Solid Edge part; units mm, degrees
sketch "Sketch1" plane through (0, 0, 0) normal (0, 0, 1) x (1, 0, 0)
  line L0 (-17.5, 30) -> (17.5, 30)
  line L1 (17.5, 30) -> (17.5, 15)
  line L2 (17.5, 15) -> (22.3, 15)
  line L3 (22.3, 0) -> (22.3, 15)
  line L4 (22.3, 0) -> (22.3, -15)
  line L5 (22.3, -15) -> (17.5, -15)
  line L6 (17.5, -30) -> (17.5, -15)
  line L7 (-17.5, -30) -> (17.5, -30)
  line L8 (-17.5, -15) -> (-17.5, -30)
  line L9 (-22.3, -15) -> (-17.5, -15)
  line L10 (-22.3, 0) -> (-22.3, -15)
  line L11 (-22.3, 0) -> (-22.3, 15)
  line L12 (-17.5, 15) -> (-22.3, 15)
  line L13 (-17.5, 15) -> (-17.5, 30)
  circle A0 centre (3.45, 14.41) radius 1.25
  circle A1 centre (-7.895, 10.99) radius 1.25
  circle A2 centre (-3.45, -14.41) radius 1.25
  circle A3 centre (7.895, -10.99) radius 1.25
extrude "ExtrudedProtrusion_6" add sketch "Sketch1" along normal blind 4.8
sketch "Sketch2" plane through (0, 0, 4.8) normal (0, 0, 1) x (1, 0, 0)
  line L0 (-19.9, 15) -> (-19.9, -15.25)
  line L1 (-19.9, -15.25) -> (-17.5, -15.25)
  line L2 (-17.5, -15.25) -> (-17.5, 15)
  line L3 (-17.5, 15) -> (-19.9, 15)
  line L4 (19.9, -15) -> (19.9, 15)
  line L5 (19.9, 15) -> (17.5, 15)
  line L6 (17.5, 15) -> (17.5, -15)
  line L7 (17.5, -15) -> (19.9, -15)
extrude "ExtrudedCutout_5" cut sketch "Sketch2" against normal blind 2.4
sketch "Sketch3" plane through (0, -0.25, 4.8) normal (0, 0, 1) x (1, 0, 0)
  line L0 (6.2615, 8.9272) -> (-10.0146, 4.0193)
  arc A0 (-13.3582, -2.2113) -> (-10.0146, 4.0193) centre (-8.5711, -0.7678) cw
  line L1 (-13.3582, -2.2113) -> (-12.7808, -4.1261)
  arc A1 (-12.7808, -4.1261) -> (-6.5502, -7.4697) centre (-7.9937, -2.6826) ccw
  line L2 (-6.5502, -7.4697) -> (9.7259, -2.5619)
  arc A2 (9.7259, -2.5619) -> (13.0695, 3.6687) centre (8.2824, 2.2252) ccw
  line L3 (13.0695, 3.6687) -> (12.4921, 5.5835)
  arc A3 (6.2615, 8.9272) -> (12.4921, 5.5835) centre (7.705, 4.1401) cw
extrude "ExtrudedCutout_7" cut sketch "Sketch3" against normal blind 5
sketch "Sketch4" plane through (0, -0.25, 4.8) normal (0, 0, 1) x (1, 0, 0)
  arc A0 (-17.5, 18.25) -> (-17.5, 15.25) centre (-17.5, 16.75) cw
  line L0 (-17.5, 15.25) -> (-17.5, 18.25)
  arc A1 (-17.5, -14.75) -> (-17.5, -17.75) centre (-17.5, -16.25) cw
  line L1 (-17.5, -14.75) -> (-17.5, -17.75)
  arc A2 (17.5, -17.75) -> (17.5, -14.75) centre (17.5, -16.25) cw
  line L2 (17.5, -14.75) -> (17.5, -17.75)
  line L3 (17.5, 15.25) -> (17.5, 18.25)
  arc A3 (17.5, 15.25) -> (17.5, 18.25) centre (17.5, 16.75) cw
extrude "Cutout1" cut sketch "Sketch4" against normal blind 5
sketch "Sketch5" plane through (0, -0.25, 0) normal (0, 0, -1) x (-1, 0, 0)
  line L0 (-1.6, 30.25) -> (-1.6, 27.2024)
  arc A0 (-1.6, 27.2024) -> (-2.725, 25.75) centre (-1.225, 25.75) ccw
  line L1 (-2.725, 25.75) -> (-2.725, 24.25)
  arc A1 (-2.725, 24.25) -> (-1.5998, 22.7976) centre (-1.225, 24.25) ccw
  arc A2 (-1.5998, 22.7976) -> (1.5998, 22.7976) centre (0, 22.7754) ccw
  arc A3 (2.725, 24.25) -> (1.5998, 22.7976) centre (1.225, 24.25) cw
  line L2 (2.725, 25.75) -> (2.725, 24.25)
  arc A4 (1.5998, 27.2024) -> (2.725, 25.75) centre (1.225, 25.75) cw
  line L3 (1.5998, 30.25) -> (1.5998, 27.2024)
  line L4 (0, 30.25) -> (1.5998, 30.25)
  line L5 (0, 30.25) -> (-1.6, 30.25)
  arc A5 (-1.5998, -22.2976) -> (1.5998, -22.2976) centre (0, -22.2754) cw
  arc A6 (2.725, -23.75) -> (1.5998, -22.2976) centre (1.225, -23.75) ccw
  line L6 (2.725, -25.25) -> (2.725, -23.75)
  arc A7 (1.5998, -26.7024) -> (2.725, -25.25) centre (1.225, -25.25) ccw
  line L7 (1.5998, -29.75) -> (1.5998, -26.7024)
  line L8 (0, -29.75) -> (1.5998, -29.75)
  line L9 (0, -29.75) -> (-1.6, -29.75)
  line L10 (-1.6, -29.75) -> (-1.6, -26.7024)
  arc A8 (-1.6, -26.7024) -> (-2.725, -25.25) centre (-1.225, -25.25) cw
  line L11 (-2.725, -25.25) -> (-2.725, -23.75)
  arc A9 (-2.725, -23.75) -> (-1.5998, -22.2976) centre (-1.225, -23.75) cw
extrude "Cutout2" cut sketch "Sketch5" against normal up to next
properties material "Polycarbonate"
Here's how the part is built. I have some questions about the finished solid (model axes, mm). A direction names the side the tool comes from. Give positions to 0.01 mm unless a question says otherwise; leave off trailing zeros. Order: outer loops, then holes, each group sorted by start corner. A loop starts at its lowest first (then second) coordinate and runs counter-clockwise, first axis right, second up. Notation, with made-up numbers: (9, 68.25) -> (57, 68.25) arc R26 ccw to (57, 104.25) -> close; hole circle Ø5 at (28.25, 78.25). An arc over 180 degrees is marked (long way). Use a Markdown table: item, result. Add a question column.
Item 1: For faces 1 (the face through (-17.5, 0, 4)), 2 (the face through (-20, -15, 2)), 3 (the face through (-10, 30, 2)), 4 (the face through (0, -6, 4.8)), 5 (the face through (10.12, 8.27, 2.43)), which set-ups out of +Z, -Z, +X, -X, +Y, -Y let a thin tool reach every point of the face, with its end or its side?
Item 2: Imagine slicing it at B-B on z = 3.95. Give the number of separate pieces and of enclosed holes in the cut face, plus the area to 3 significant figures.
Item 3: I need wall thicknesses on line 1 (X direction, y = -24.5, z = 2) (3 decimals); line 2 (Y direction, x = 8.5, z = 3.75); line 3 (Y direction, x = -3.45, z = 2). Which ranges of each line are inside material? Lowest first, please.
Item 4: Imagine slicing it at A-A on y = -10.99. Please give me the cut outline in (x, z) (3 decimals), plus the area to 3 significant figures.
Item 5: Will these pins go through, and if not, where does the flat tip stop? pin 1 (3 mm diameter, centred on x = -3.45, y = -14.41, fed in from -Z); pin 2 (0.9 mm diameter, centred on y = -28, z = 1.5, fed in from +X); pin 3 (0.9 mm diameter, centred on y = 28, z = 3, fed in from -X).
Item 6: Imagine slicing it at D-D on x = 8. Please give me the cut outline in (y, z).
Item 7: Imagine slicing it at C-C on x = 0.5. Please give me the cut outline in (y, z).
Item 8: If we mould it in two halves opening along X, with no side actions, what happens to faces 6 (the face through (21, 0, 4.8)), 7 (the face through (-1.76, 6.26, 2.43)), 8 (the face through (16, 16.5, 2.4))? For each: pulls with the +X half, pulls with the -X half, needs draft (parallel to the pull), parting line crosses it, or undercut.
Data:
| question | item | result |
|---|---|---|
| 1 | face 1 | +Z, +Y, -Y |
| 1 | face 2 | +Z, -Z, -X, -Y |
| 1 | face 3 | +Z, -Z, +X, -X, +Y |
| 1 | face 4 | +Z, +X, -X, +Y, -Y |
| 1 | face 5 | +Z, -Z |
| 2 | separate pieces | 3 |
| 2 | enclosed holes | 5 |
| 2 | area | 1,840 mm² |
| 3 | line 1 | x = -17.5 to -2.725, 2.725 to 17.5 |
| 3 | line 2 | y = -30 to -12.08, -9.9 to -3.18, 8.83 to 30 |
| 3 | line 3 | y = -30 to -15.66, -13.16 to -6.78, 5.75 to 30 |
| 4 | outline | (-22.3, 0) -> (6.645, 0) -> (6.645, 4.8) -> (-17.5, 4.8) -> (-17.5, 2.4) -> (-19.9, 2.4) -> (-19.9, 4.8) -> (-22.3, 4.8) -> close; (9.145, 0) -> (22.3, 0) -> (22.3, 4.8) -> (19.9, 4.8) -> (19.9, 2.4) -> (17.5, 2.4) -> (17.5, 4.8) -> (9.145, 4.8) -> close |
| 4 | area | 191 mm² |
| 5 | pin 1 | stops at z = 0 |
| 5 | pin 2 | stops at x = 17.5 |
| 5 | pin 3 | stops at x = -17.5 |
| 6 | outline | (-30, 0) -> (-12.24, 0) -> (-12.24, 4.8) -> (-30, 4.8) -> close; (-9.74, 0) -> (-3.33, 0) -> (-3.33, 4.8) -> (-9.74, 4.8) -> close; (8.88, 0) -> (30, 0) -> (30, 4.8) -> (8.88, 4.8) -> close |
| 7 | outline | (-21.01, 0) -> (-5.59, 0) -> (-5.59, 4.8) -> (-21.01, 4.8) -> close; (6.94, 0) -> (21.01, 0) -> (21.01, 4.8) -> (6.94, 4.8) -> close |
| 8 | face 6 | needs draft |
| 8 | face 7 | undercut |
| 8 | face 8 | pulls with the +X half |
